```python
from build123d import *

# Parameters (mm, degrees)
ESBO_O1_R                = 2
ESBO_O1_R_2              = 5.5
RESSALTO_EXTRUS_O1_DEPTH = 9.7
ESBO_O2_R                = 8.5
ESBO_O2_R_2              = 2.8
RESSALTO_EXTRUS_O2_DEPTH = 5.3


with BuildPart() as part:
    # Esboço1 → Ressalto-extrusão1 (new body)
    with BuildSketch(Plane.XY):
        with BuildLine():
            Line((-3.631457669, -11.855371335), (0.071926714, -42.412329846))
            ThreePointArc((0.071926714, -42.412329846), (6.924703408, -48.086484209), (12.957802317, -41.547501589))
            Line((12.957802317, -41.547501589), (12.397968723, 0.166390596))
            ThreePointArc((12.397968723, 0.166390596), (-7.439329204, 9.919359621), (-3.631457669, -11.855371335))
        make_face()
        with Locations((6.491667521, -41.634282258)):
            Circle(ESBO_O1_R, mode=Mode.SUBTRACT)
        Circle(ESBO_O1_R_2, mode=Mode.SUBTRACT)
    extrude(amount=RESSALTO_EXTRUS_O1_DEPTH)

    # Esboço2 → Ressalto-extrusão2 (add)
    with BuildSketch(Plane.XY.offset(9.7)):
        Circle(ESBO_O2_R)
        Circle(ESBO_O2_R_2, mode=Mode.SUBTRACT)
    extrude(amount=RESSALTO_EXTRUS_O2_DEPTH)


solid = part.part
```
Geometry check sheet. Reference: the model listing, model coordinates, mm. A direction names the side the tool comes from. Round coordinates to 2 decimals unless told otherwise and drop trailing zeros. Loops run counter-clockwise (first coordinate to the right, second up) from the corner with the lowest first, then second, coordinate; pieces in that order, holes last. Notation, with made-up numbers: (-25.75, -17.75) - (-2.75, -17.75) arc R24 ccw to (-2.75, 12.25) - close; hole circle Ø6 at (44.5, 76). An arc over 180 degrees is marked (long way). Write each question's results on one line, items separated by ' | '. Start each with the question number.
Q1. Cross-section at A-A on z = 12.5. Enter the section's corners in (x, y), and give its area (3 significant figures).
Q2. Release check for a two-part mould opening along Y. For faces 3 (the flat face through (4, 0, 15)), 4 (the cylindrical face through (-1.19, -5.37, 4.78)), 5 (the cylindrical face through (4.57, 7.167, 12.313)) record: +Y half, -Y half, draft (parallel to the pull), parting line (faces both ways), or undercut.
Q3. Access from +Z, -Z, +X, -X, +Y, -Y to the whole of each face (thin tool, end or side, straight path). Record for faces 1 (the cylindrical face through (7.41, -43.41, 4.78)), 2 (the flat face through (-3, 1, 9.7)).
Q4. Thickness scan on line 1 (Y direction, x = 0, z = 12.7); line 2 (Z direction, x = 3.75, y = -35); line 3 (Y direction, x = 5, z = 6.5). Record the ranges inside material, lowest first. Write a range as [from, to].
Q5. Cross-section at B-B on x = -1.75. Enter the section's corners in (y, z).
Q6. Cross-section at C-C on y = 6.5. Enter the section's corners in (x, z).
Q7. Gauge pin test, flat ends, axial feed: P1, Ø7.5, axis at x = 2.5, y = -19, coming from the +Z side; P2, Ø3.5, axis at x = 2.5, y = -1.5, coming from the -Z side; P3, Ø6, axis at x = -4, z = 4.5, coming from the +Y side; P4, Ø2.5, axis at x = 6.49, y = -41.63, coming from the -Z side. Record the tip position at first contact, or that the pin passes through.
Q8. Cross-section at D-D on z = 8.5. Enter the section's corners in (x, y).
Answers below:
1) outline: circle Ø17 at (0, 0); hole circle Ø5.6 at (0, 0) | area: 202 mm²
2) face 3: draft | face 4: undercut | face 5: parting line
3) face 1: +Z, -Z | face 2: -Z
4) line 1: y = [-8.5, -2.8], [2.8, 8.5] | line 2: z = [0, 9.7] | line 3: y = [-47.93, -42.97], [-40.3, -2.29], [2.29, 11.35]
5) outline: (-27.38, 0) - (-5.21, 0) - (-5.21, 9.7) - (-2.19, 9.7) - (-2.19, 15) - (-8.32, 15) - (-8.32, 9.7) - (-27.38, 9.7) - close; (2.19, 9.7) - (5.21, 9.7) - (5.21, 0) - (12.27, 0) - (12.27, 9.7) - (8.32, 9.7) - (8.32, 15) - (2.19, 15) - close
6) outline: (-10.56, 0) - (10.56, 0) - (10.56, 9.7) - (5.48, 9.7) - (5.48, 15) - (-5.48, 15) - (-5.48, 9.7) - (-10.56, 9.7) - close
7) P1: stops at z = 9.7 | P2: stops at z = 9.7 | P3: stops at y = 12.36 | P4: passes through
8) outline: (-3.63, -11.86) - (0.07, -42.41) arc R6.47 ccw to (12.96, -41.55) - (12.4, 0.17) arc R12.4 ccw (long way) to start; hole circle Ø11 at (0, 0); hole circle Ø4 at (6.49, -41.63)
